CAD build for the part. Positions are in the model's coordinates, mm. A direction names the side the tool comes from. Round coordinates to 2 decimals unless told otherwise and drop trailing zeros. Order: outer loops, then holes, each group sorted by start corner. A loop starts at its lowest first (then second) coordinate and runs counter-clockwise, first axis right, second up. Notation, with made-up numbers: (-9, -21.75) -> (10, -21.75) arc R21 cw to (10, -1.75) -> close; hole circle Ø4 at (2.25, -29). An arc over 180 degrees is marked (long way). Return JSON: item names as keys, results as strings. Group by question number.
Q1. Probe line 1 along Y through (x, z) = (0, -6); line 2 along Y through (x, z) = (0, 2). List the from-to ranges inside material, lowest first.
Q2. Mould opens along X. For faces 4 (the conical face through (-18.045, -5.683, -3.085)), 5 (the cylindrical face through (-20.97, 8.69, 3.08)), 6 (the flat face through (-5, 20, -12)) say: +X half, -X half, draft (parallel to the pull), parting line (faces both ways), or undercut.
Q3. Cut at A-A (y = 0). Write the cut outline in (x, z).
Q4. Cut at D-D (z = 6.75). Write the cut outline in (x, y).
Q5. Which spindle directions (+Z, -Z, +X, -X, +Y, -Y) get a long thin tool onto all of the face, cutting with end or side? Do faces 1 (the cylindrical face through (2.708, -20.623, -7.706)), 2 (the cylindrical face through (16.427, 12.596, 4.056)), 3 (the flat face through (18.4, 10, 8)). Say none if no direction does.
Q6. Cut at C-C (z = -8.25). Write the cut outline in (x, y), then the cut area to 3 significant figures.
Q7. Flat gauge pins, fed straight in: pin 1 (10 mm diameter, centred on x = -5.5, z = 1.5, fed in from +Y); pin 2 (3 mm diameter, centred on y = 14, z = 0, fed in from +X); pin 3 (2 mm diameter, centred on x = 9.5, z = -7.5, fed in from +Y). Where does each tip first touch, or does it go through?
from build123d import *

# Parameters (mm, degrees)
F2_SIZE = 1.5


with BuildPart() as f1:
    # F0 (on Front) → F1 (revolve)
    with BuildSketch(Plane.XZ):
        Polygon((-20.7, 8), (-22.7, 8), (-22.7, -1.696607), (-20.8, -3.290897), (-20.8, -12), (-18.8, -12), (-18.8, -3.290897), (-20.7, 0), align=None)
    revolve(axis=Axis((0, 0, 4.153483), (0, 0, 1)))

    # F2
    f2_edges = [f1.edges().sort_by_distance(p)[0] for p in [
        (18.8, 0, -12),
    ]]
    chamfer(f2_edges, length=F2_SIZE)


solid = f1.part
Solution:
{
 "1": {"line 1": "y = -20.8 to -18.8, 18.8 to 20.8", "line 2": "y = -22.7 to -20.7, 20.7 to 22.7"},
 "2": {"face 4": "undercut", "face 5": "parting line", "face 6": "draft"},
 "3": {"outline": "(-22.7, -1.7) -> (-20.8, -3.29) -> (-20.8, -12) -> (-20.3, -12) -> (-18.8, -10.5) -> (-18.8, -3.29) -> (-20.7, 0) -> (-20.7, 8) -> (-22.7, 8) -> close; (18.8, -10.5) -> (20.3, -12) -> (20.8, -12) -> (20.8, -3.29) -> (22.7, -1.7) -> (22.7, 8) -> (20.7, 8) -> (20.7, 0) -> (18.8, -3.29) -> close"},
 "4": {"outline": "circle Ø45.4 at (0, 0); hole circle Ø41.4 at (0, 0)"},
 "5": {"face 1": "-Z", "face 2": "+Z", "face 3": "+Z, +X, -X, +Y, -Y"},
 "6": {"outline": "circle Ø41.6 at (0, 0); hole circle Ø37.6 at (0, 0)", "area": "249 mm²"},
 "7": {"pin 1": "stops at y = 22.69", "pin 2": "stops at x = 18.95", "pin 3": "stops at y = 18.98"}
}
